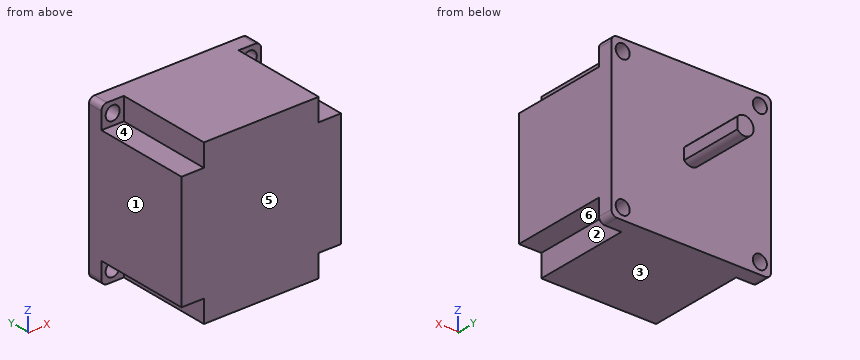
Autodesk Inventor part; units mm, degrees
ref_plane "YZ Plane" through (0, 0, 0) normal (1, 0, 0) x (0, 1, 0)
ref_plane "XZ Plane" through (0, 0, 0) normal (0, 1, 0) x (-1, 0, 0)
ref_plane "XY Plane" through (0, 0, 0) normal (0, 0, 1) x (1, 0, 0)
sketch "Sketch1" plane through (0, 0, 0) normal (0, 1, 0) x (-1, 0, 0)
  line L0 (-28.5, 28.5) -> (28.5, 28.5)
  line L1 (28.5, 28.5) -> (28.5, -28.5)
  line L2 (28.5, -28.5) -> (-28.5, -28.5)
  line L3 (-28.5, -28.5) -> (-28.5, 28.5)
  line L4 (-28.5, 28.5) -> (28.5, -28.5) construction
  line L5 (28.5, 28.5) -> (-28.5, -28.5) construction
  line L6 (28.5, -28.5) -> (20.5, -28.5)
  line L7 (20.5, -28.5) -> (20.5, -20.5)
  line L8 (20.5, -20.5) -> (28.5, -20.5)
  line L9 (28.5, -20.5) -> (28.5, -28.5)
  line L10 (-28.5, -28.5) -> (-22.5, -28.5)
  line L11 (-22.5, -28.5) -> (-22.5, -20.5)
  line L12 (-22.5, -20.5) -> (-28.5, -20.5)
  line L13 (-28.5, -20.5) -> (-28.5, -28.5)
  line L14 (-28.5, 28.5) -> (-20.5, 28.5)
  line L15 (-20.5, 28.5) -> (-20.5, 20.5)
  line L16 (-20.5, 20.5) -> (-28.5, 20.5)
  line L17 (-28.5, 20.5) -> (-28.5, 28.5)
  line L18 (28.5, 28.5) -> (20.5, 28.5)
  line L19 (20.5, 28.5) -> (20.5, 20.5)
  line L20 (20.5, 20.5) -> (28.5, 20.5)
  line L21 (28.5, 20.5) -> (28.5, 28.5)
  line L22 (-28.5, -28.5) -> (-20.5, -28.5)
  line L23 (-20.5, -28.5) -> (-20.5, -20.5)
  line L24 (-20.5, -20.5) -> (-28.5, -20.5)
  line L25 (-28.5, -20.5) -> (-28.5, -28.5)
  point P0 (0, 0)
  point P1 (28.5, 20.5)
  point P2 (20.5, 28.5)
  point P3 (-20.5, 28.5)
  point P4 (-28.5, 20.5)
  point P5 (-28.5, -20.5)
  point P6 (20.5, -28.5)
  dimension "d0" = 57
  dimension "d1" = 57
  dimension "d2" = 8
  dimension "d3" = 8
  dimension "d4" = 6
  dimension "d5" = 8
  dimension "d6" = 8
  dimension "d7" = 8
  dimension "d8" = 8
  dimension "d9" = 8
  dimension "d19" = 8
  dimension "d20" = 8
extrude "Extrusion1" add sketch "Sketch1" along normal blind 40 contours L0 L19 L20 L1 L8 L7 L2 L23 L24 L12 L3 L16 L15
sketch "Sketch2" plane through (0, 40, 0) normal (0, 1, 0) x (1, 0, 0)
  line L0 (-20.5, -20.5) -> (-20.5, -28.5)
  line L1 (-20.5, -28.5) -> (20.5, -28.5)
  line L2 (20.5, -28.5) -> (20.5, -20.5)
  line L3 (20.5, -20.5) -> (28.5, -20.5)
  line L4 (28.5, -20.5) -> (28.5, 20.5)
  line L5 (28.5, 20.5) -> (20.5, 20.5)
  line L6 (20.5, 28.5) -> (-20.5, 28.5)
  line L7 (-20.5, 28.5) -> (-20.5, 20.5)
  line L8 (-20.5, 20.5) -> (-28.5, 20.5)
  line L9 (-28.5, 20.5) -> (-28.5, -20.5)
  line L10 (-28.5, -20.5) -> (-20.5, -20.5)
  circle A0 centre (0, 0) radius 3.25
  line L11 (20.5, 20.5) -> (20.5, 28.5)
  line L12 (-3.25, 0) -> (2.55, 0)
  line L13 (2.55, 2.0149) -> (2.55, -2.0149)
  dimension "d12" = 6.5
  dimension "d24" = 5.8
extrude "Extrusion2" add sketch "Sketch2" along normal blind 23 contours L13 L12 A0 | A0 L12 L13
sketch "Sketch3" plane through (0, 40, 0) normal (0, 1, 0) x (1, 0, 0)
  arc A0 (2.55, 2.0149) -> (2.55, -2.0149) centre (0, 0) ccw
  line L0 (-20.5, -20.5) -> (-20.5, -28.5)
  line L1 (-20.5, -28.5) -> (20.5, -28.5)
  line L2 (20.5, -28.5) -> (20.5, -20.5)
  line L3 (20.5, -20.5) -> (28.5, -20.5)
  line L4 (28.5, -20.5) -> (28.5, 20.5)
  line L5 (28.5, 20.5) -> (20.5, 20.5)
  line L6 (20.5, 28.5) -> (-20.5, 28.5)
  line L7 (-20.5, 28.5) -> (-20.5, 20.5)
  line L8 (-20.5, 20.5) -> (-28.5, 20.5)
  line L9 (-28.5, 20.5) -> (-28.5, -20.5)
  line L10 (-28.5, -20.5) -> (-20.5, -20.5)
  line L11 (-28.5, -28.5) -> (28.5, -28.5)
  line L12 (28.5, -28.5) -> (28.5, 28.5)
  line L13 (28.5, 28.5) -> (-28.5, 28.5)
  line L14 (-28.5, 28.5) -> (-28.5, -28.5)
  line L15 (20.5, 20.5) -> (20.5, 28.5)
  line L16 (2.55, 2.0149) -> (2.55, -2.0149)
  point P0 (-28.5, 20.5)
  point P1 (-28.5, -20.5)
  point P2 (-20.5, -28.5)
  point P3 (20.5, -28.5)
  point P4 (28.5, -20.5)
  point P5 (28.5, 20.5)
extrude "Extrusion3" add sketch "Sketch3" against normal blind 5.4 contours L16 A0 | L10 L9 L8 L7 L6 L15 L5 L4 L3 L2 L1 L0 | L0 L11 L14 L10 | L2 L3 L12 L11 | L14 L13 L7 L8 | L5 L15 L13 L12
fillet "Fillet1" radius 2 4 edges at (28.5, 37.3, 28.5) (-28.5, 37.3, 28.5) (-28.5, 37.3, -28.5) (28.5, 37.3, -28.5)
sketch "Sketch4" plane through (0, 40, 0) normal (0, 1, 0) x (1, 0, 0)
  line L0 (-20.5, 20.5) -> (-28.5, 20.5)
  line L1 (-20.5, 28.5) -> (-20.5, 20.5)
  line L2 (20.5, 28.5) -> (-20.5, 28.5)
  line L3 (28.5, 20.5) -> (20.5, 20.5)
  line L4 (28.5, -20.5) -> (28.5, 20.5)
  line L5 (20.5, -20.5) -> (28.5, -20.5)
  line L6 (20.5, -28.5) -> (20.5, -20.5)
  line L7 (-20.5, -28.5) -> (20.5, -28.5)
  line L8 (-20.5, -20.5) -> (-20.5, -28.5)
  line L9 (-28.5, -20.5) -> (-20.5, -20.5)
  line L10 (-28.5, 20.5) -> (-28.5, -20.5)
  line L11 (20.5, -20.5) -> (28.5, -20.5)
  line L12 (20.5, -20.5) -> (28.5, -20.5)
  line L13 (28.5, -20.5) -> (28.5, -28.5)
  line L14 (28.5, -28.5) -> (20.5, -28.5)
  line L15 (20.5, -28.5) -> (20.5, -20.5)
  line L16 (20.5, 20.5) -> (20.5, 28.5)
  circle A0 centre (24.5, -24.5) radius 2.5
  point P0 (0, 0)
  dimension "d21" = 5
extrude "Extrusion4" cut sketch "Sketch4" against normal blind 40 contours A0
ref_plane "Work Plane1" through (0, 0, 20.5) normal (1, 0, 0) x (0, 0, -1)
ref_plane "Work Plane2" through (20.5, 0, 0) normal (0, 0, -1) x (-1, 0, 0)
mirror "Mirror1" about plane through (0, 0, 20.5) normal (1, 0, 0) of "Extrusion4"
mirror "Mirror2" about plane through (20.5, 0, 0) normal (0, 0, -1) of "Extrusion4", "Mirror1"
properties part number "Motor"
Geometry: final body of the model. Coordinates: model frame, mm. Face numbers are marked on the shaded views. A direction names the side the tool comes from. Give positions to 0.01 mm unless a question says otherwise; leave off trailing zeros. Loops run counter-clockwise (first coordinate to the right, second up) from the corner with the lowest first, then second, coordinate; pieces in that order, holes last. Notation, with made-up numbers: (68.25, 85.5) -> (102.25, 85.5) arc R23 cw to (102.25, 118.5) -> close; hole circle Ø11 at (-39, -30.75). An arc over 180 degrees is marked (long way). Return JSON: item names as keys, results as strings.
Item 1: Section C-C, the plane x = 0. Output: boundary loops of the cut face in (y, z).
Filled in:
{"outline": "(0, -28.5) -> (40, -28.5) -> (40, -3.25) -> (63, -3.25) -> (63, 3.25) -> (40, 3.25) -> (40, 28.5) -> (0, 28.5) -> close"}
Item 2: Section A-A, the plane x = -24.5. Output: boundary loops of the cut face in (y, z), plus the area to 3 significant figures.
Filled in:
{"outline": "(0, -20.5) -> (34.6, -20.5) -> (34.6, -22) -> (40, -22) -> (40, 22) -> (34.6, 22) -> (34.6, 20.5) -> (0, 20.5) -> close; (34.6, -28.5) -> (40, -28.5) -> (40, -27) -> (34.6, -27) -> close; (34.6, 27) -> (40, 27) -> (40, 28.5) -> (34.6, 28.5) -> close", "area": "1,670 mm^2"}
Item 3: Mould query, pull axis X, two halves, no side actions, for the marked faces 1, 2 and 3. Classes: released by +X, released by -X, zero draft, split by the parting line, or undercut.
Filled in:
{"face 1": "released by -X", "face 2": "released by +X", "face 3": "zero draft"}
Item 4: Pin query (flat end, axial travel): P1, Ø2.5, axis at x = -23.5, z = 24.5, coming from the -Y side; P2, Ø12, axis at x = 12.5, z = -5.5, coming from the +Y side; P3, Ø6.5, axis at x = -24.5, y = 23.5, coming from the -Z side; P4, Ø2.5, axis at x = 24, z = -22.5, coming from the -Y side. Return the tip coordinate at first contact, or that it passes through.
Filled in:
{"P1": "through", "P2": "y = 40", "P3": "z = -20.5", "P4": "y = 34.6"}
Item 5: Access query for the marked faces 4, 5 and 6. Directions: +Z, -Z, +X, -X, +Y, -Y. A direction counts if a zero-diameter tool reaches every point of the face in a straight line with its end or side. Return the directions, or none.
Filled in:
{"face 4": "+Z, -X, -Y", "face 5": "+Z, -Z, +X, -X, -Y", "face 6": "-Z, +X, -Y"}
Item 6: Section B-B, the plane z = 24.5. Output: boundary loops of the cut face in (x, y).
Filled in:
{"outline": "(-28.5, 34.6) -> (-27, 34.6) -> (-27, 40) -> (-28.5, 40) -> close; (-22, 34.6) -> (-20.5, 34.6) -> (-20.5, 0) -> (20.5, 0) -> (20.5, 34.6) -> (22, 34.6) -> (22, 40) -> (-22, 40) -> close; (27, 34.6) -> (28.5, 34.6) -> (28.5, 40) -> (27, 40) -> close"}
Item 7: Line query: line 1 (X direction, y = 38.15, z = 24.5); line 2 (Z direction, x = -24, y = 38). Output: solid intervals per line, ascending.
Filled in:
{"line 1": "-28.5 to -27, -22 to 22, 27 to 28.5", "line 2": "-28.5 to -26.95, -22.05 to 22.05, 26.95 to 28.5"}
Item 8: Section D-D, the plane y = 22. Output: boundary loops of the cut face in (x, z), plus the area to 3 significant figures.
Filled in:
{"outline": "(-28.5, -20.5) -> (-20.5, -20.5) -> (-20.5, -28.5) -> (20.5, -28.5) -> (20.5, -20.5) -> (28.5, -20.5) -> (28.5, 20.5) -> (20.5, 20.5) -> (20.5, 28.5) -> (-20.5, 28.5) -> (-20.5, 20.5) -> (-28.5, 20.5) -> close", "area": "2,990 mm^2"}
